For this review, use the dimensioned drawing (mm, ordinates from the lowest corner) and the shaded views. A direction names the side the tool comes from. Give positions to 0.01 mm unless a question says otherwise; leave off trailing zeros. Order: outer loops, then holes, each group sorted by start corner. A loop starts at its lowest first (then second) coordinate and runs counter-clockwise, first axis right, second up. Notation, with made-up numbers: (70.25, 72.5) - (123.25, 72.5) arc R16 cw to (123.25, 76.5) - close; hole circle Ø11 at (-14.75, 64). An arc over 180 degrees is marked (long way). Use a Markdown table: item, result. Add a question column.
1) We need section C-C on y = 78. Write out the cut boundary in (x, z).
2) Machinability: for the marked faces 4 and 5, which of the approach directions +Z, -Z, +X, -X, +Y, -Y give a long, thin tool a straight path to every point of the face, cutting with its end or side? Answer none if there is none.
3) Wall thickness on L1, parallel to X at y = 145, z = 737: over which ranges is the line inside the solid? List them lowest first.
4) We need section A-A on x = 1336.5. Write out the cut boundary in (y, z).
5) Mouldability with a two-part tool opening along X and no side actions: class the marked faces 1, 2 and 3 as released by +X, released by -X, zero draft, split by the parting line, or undercut.
6) We need section B-B on z = 864. Write out the cut boundary in (x, y).
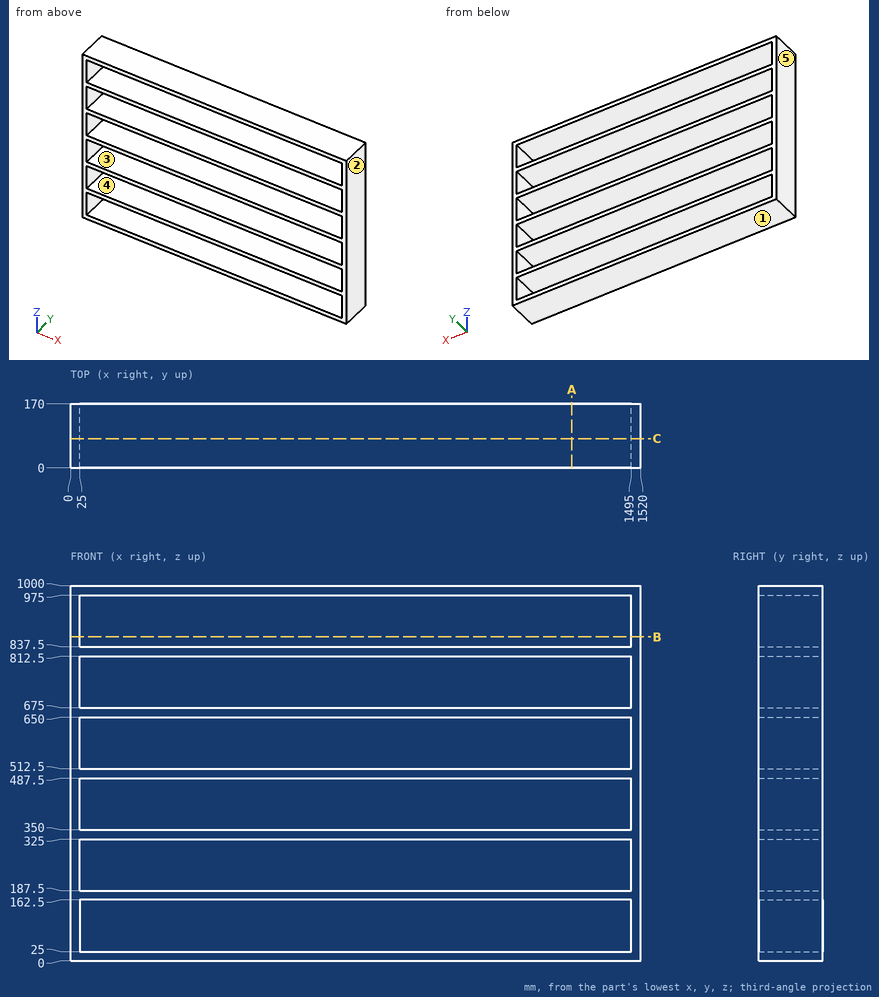
Checked values:
| question | item | result |
|---|---|---|
| 1 | outline | (0, 0) - (1520, 0) - (1520, 1000) - (0, 1000) - close; hole (25, 25) - (1495, 25) - (1495, 162.5) - (25, 162.5) - close; hole (25, 187.5) - (1495, 187.5) - (1495, 325) - (25, 325) - close; hole (25, 350) - (1495, 350) - (1495, 487.5) - (25, 487.5) - close; hole (25, 512.5) - (1495, 512.5) - (1495, 650) - (25, 650) - close; hole (25, 675) - (1495, 675) - (1495, 812.5) - (25, 812.5) - close; hole (25, 837.5) - (1495, 837.5) - (1495, 975) - (25, 975) - close |
| 2 | face 4 | +Y, -Y |
| 2 | face 5 | +Z, -Z, -X, +Y, -Y |
| 3 | L1 | 0 to 25, 1495 to 1520 |
| 4 | outline | (0, 0) - (170, 0) - (170, 25) - (0, 25) - close; (0, 162.5) - (170, 162.5) - (170, 187.5) - (0, 187.5) - close; (0, 325) - (170, 325) - (170, 350) - (0, 350) - close; (0, 487.5) - (170, 487.5) - (170, 512.5) - (0, 512.5) - close; (0, 650) - (170, 650) - (170, 675) - (0, 675) - close; (0, 812.5) - (170, 812.5) - (170, 837.5) - (0, 837.5) - close; (0, 975) - (170, 975) - (170, 1000) - (0, 1000) - close |
| 5 | face 1 | zero draft |
| 5 | face 2 | released by +X |
| 5 | face 3 | undercut |
| 6 | outline | (0, 0) - (25, 0) - (25, 170) - (0, 170) - close; (1495, 0) - (1520, 0) - (1520, 170) - (1495, 170) - close |
